from build123d import *

# Parameters (mm, degrees)
F1_DEPTH = 6.35
F3_DEPTH = 3.175
F5_DEPTH = 3.175


with BuildPart() as f1:
    # F0 (on Top) → F1 (new body)
    with BuildSketch(Plane.XY):
        Polygon((-177.8, 0), (0, 0), (0, 139.7), (-25.4, 139.7), (-25.4, 79.375), (-25.4, 25.4), (-79.375, 25.4), (-177.8, 25.4), align=None)
        Polygon((-79.375, 28.575), (-79.375, 25.4), (-25.4, 25.4), (-25.4, 79.375), (-28.575, 79.375), (-28.575, 28.575), align=None)
    extrude(amount=F1_DEPTH)

    # F2 (on face) → F3 (cut)
    with BuildSketch(Plane.XY.offset(6.35)):
        Polygon((0, 139.7), (-12.7, 139.7), (-12.7, 12.7), (-177.8, 12.7), (-177.8, 0), (-12.7, 0), (0, 0), (0, 12.7), align=None)
    extrude(amount=-F3_DEPTH, mode=Mode.SUBTRACT)

    # F4 (on face) → F5 (cut)
    with BuildSketch(Plane.XY.offset(6.35)):
        Polygon((-28.575, 28.575), (-79.375, 28.575), (-79.375, 25.4), (-25.4, 25.4), (-25.4, 79.375), (-28.575, 79.375), align=None)
    extrude(amount=-F5_DEPTH, mode=Mode.SUBTRACT)


solid = f1.part
Model file for the job. Use its own axes, mm. Coordinates: 2 decimals unless noted, no trailing zeros. Order: outer loops, then holes, each group sorted by start corner. A loop starts at its lowest first (then second) coordinate and runs counter-clockwise, first axis right, second up. Notation, with made-up numbers: M -39.75,48.5 L -4.75,48.5 A20 cw -4.75,57.5 Z; hole C -25.75,53.25 d10. An arc over 180 degrees is marked long. Return JSON: item names as keys, results as strings.
1. Saw through at D-D (y = 38.5). Give the cut face in (x, z) (3 decimals), and give its area (3 significant figures).
Ans:
{"outline": "M -28.575,0 L 0,0 L 0,3.175 L -12.7,3.175 L -12.7,6.35 L -25.4,6.35 L -25.4,3.175 L -28.575,3.175 Z", "area": "131 mm^2"}
2. Saw through at B-B (y = 93). Give the cut face in (x, z) (3 decimals).
Ans:
{"outline": "M -25.4,0 L 0,0 L 0,3.175 L -12.7,3.175 L -12.7,6.35 L -25.4,6.35 Z"}
3. Saw through at A-A (z = 1.75). Give the cut face in (x, y) (3 decimals), and give its area (3 significant figures).
Ans:
{"outline": "M -177.8,0 L 0,0 L 0,139.7 L -25.4,139.7 L -25.4,79.375 L -28.575,79.375 L -28.575,28.575 L -79.375,28.575 L -79.375,25.4 L -177.8,25.4 Z", "area": "7,750 mm^2"}
4. Drill centre lines: probe 1 along Y at (x, z) = (-156, 0.5); probe 2 along X at (y, z) = (112.5, 5); probe 3 along Y at (x, z) = (-22.5, 5.25). Where is each one in solid material? Low to high.
Ans:
{"probe 1": "0 to 25.4", "probe 2": "-25.4 to -12.7", "probe 3": "12.7 to 139.7"}
5. Flat gauge pins, fed straight in: pin 1 (1.6 mm diameter, centred on x = -26.5, z = 2, fed in from +Y) (3 decimals); pin 2 (2 mm diameter, centred on x = -39, z = 2.5, fed in from -Y); pin 3 (1 mm diameter, centred on x = -58.5, z = 2.5, fed in from +Y) (3 decimals); pin 4 (1.9 mm diameter, centred on y = 103, z = 1.5, fed in from -X). Where does each tip first touch, or does it go through?
Ans:
{"pin 1": "y = 79.375", "pin 2": "y = 0", "pin 3": "y = 28.575", "pin 4": "x = -25.4"}
6. Saw through at C-C (x = -41.5). Give the cut face in (y, z) (3 decimals).
Ans:
{"outline": "M 0,0 L 28.575,0 L 28.575,3.175 L 25.4,3.175 L 25.4,6.35 L 12.7,6.35 L 12.7,3.175 L 0,3.175 Z"}
